```python
from build123d import *

# Parameters (mm, degrees)
SKETCH_1_R          = 21
SKETCH_1_R_2        = 10
EXTRUDE_1_DEPTH     = 36
SKETCH_1_R_3        = 16
EXTRUDE_1_2_DEPTH   = 36
SKETCH_2_W          = 150
SKETCH_2_H          = 5
EXTRUDE_3_DEPTH     = 5
SKETCH_3_W          = 150
SKETCH_3_H          = 5
EXTRUDE_4_DEPTH     = 5
EXTRUDE_5_DEPTH     = 5
EXTRUDE_START       = -3
SKETCH_7_R          = 16
EXTRUDE_7_DEPTH     = 30
SKETCH_8_R          = 0.9
CUT_EXTRUDE_1_DEPTH = 8
EXTRUDE_START_2     = -7
SKETCH_10_R         = 18.243216987
SKETCH_10_R_2       = 11
EXTRUDE_8_DEPTH     = 22


with BuildPart() as part:
    # Sketch 1 → Extrude 1 (new body)
    with BuildSketch(Plane(origin=(0, 0, 0), x_dir=(1, 0, 0), z_dir=(0, 1, 0))):
        with Locations((68.910572273, -5.294054995)):
            Circle(SKETCH_1_R)
        with Locations((68.910572273, -5.294054995)):
            Circle(SKETCH_1_R_2, mode=Mode.SUBTRACT)
    extrude(amount=EXTRUDE_1_DEPTH)



with BuildPart() as body_2:
    # Sketch 1 → Extrude 1 2 (new body)
    with BuildSketch(Plane(origin=(0, 0, 0), x_dir=(1, 0, 0), z_dir=(0, 1, 0))):
        with Locations((-81.089427727, -5.294054995)):
            Circle(SKETCH_1_R)
        with Locations((-81.089427727, -5.294054995)):
            Circle(SKETCH_1_R_3, mode=Mode.SUBTRACT)
    extrude(amount=EXTRUDE_1_2_DEPTH)


with BuildPart() as part_1:
    add(part.part)

    add(body_2.part)  # Extrude 3 merges body 2
    # Sketch 2 → Extrude 3 (add)
    with BuildSketch(Plane(origin=(0, 36, 0), x_dir=(1, 0, 0), z_dir=(0, 1, 0))):
        with Locations((-6.089427727, -23.794054995)):
            Rectangle(SKETCH_2_W, SKETCH_2_H)
        with Locations((-6.089427727, 13.205945005)):
            Rectangle(SKETCH_2_W, SKETCH_2_H)
    extrude(amount=-EXTRUDE_3_DEPTH)

    # Sketch 3 → Extrude 4 (add)
    with BuildSketch(Plane.XZ):
        with Locations((-6.089427727, -13.205945005)):
            Rectangle(SKETCH_3_W, SKETCH_3_H)
        with Locations((-6.089427727, 23.794054995)):
            Rectangle(SKETCH_3_W, SKETCH_3_H)
    extrude(amount=-EXTRUDE_4_DEPTH)

    # Sketch 4 → Extrude 5 (add)
    with BuildSketch(Plane.XZ):
        Polygon((-36.788692473, 8.113223678), (-7.244877213, 23.511020598), (-6.089427727, 21.294054995), (-4.933978242, 23.511020598), (24.609837018, 8.113223678), (54.153652279, 23.511020598), (56.46455125, 19.077089392), (30.018987378, 5.294054995), (56.46455125, -8.488979402), (54.153652279, -12.922910608), (24.609837018, 2.474886312), (-4.933978242, -12.922910608), (-7.244877213, -12.922910608), (-36.788692473, 2.474886312), (-66.332507733, -12.922910608), (-68.643406704, -8.488979402), (-42.197842833, 5.294054995), (-68.643406704, 19.077089392), (-66.332507733, 23.511020598), align=None)
        Polygon((-31.379542113, 5.294054995), (-8.589427727, -6.583813521), (-8.589427727, 17.17192351), align=None, mode=Mode.SUBTRACT)
        Polygon((-3.589427727, -6.583813521), (19.200686659, 5.294054995), (-3.589427727, 17.17192351), align=None, mode=Mode.SUBTRACT)
    extrude_5 = extrude(amount=-EXTRUDE_5_DEPTH)

    # Sketch 7 → Extrude 7 (add)
    with BuildSketch(Plane(origin=(0, 36, 0), x_dir=(1, 0, 0), z_dir=(0, 1, 0)).offset(EXTRUDE_START)):
        with Locations((68.910572273, -5.294054995)):
            Circle(SKETCH_7_R)
    extrude(amount=-EXTRUDE_7_DEPTH)

    # Sketch 8 → Cut-Extrude 1 (cut)
    with BuildSketch(Plane(origin=(0, 33, 0), x_dir=(1, 0, 0), z_dir=(0, 1, 0))):
        with Locations((76.910572273, -5.294054995)):
            Circle(SKETCH_8_R)
        with Locations((68.910572273, 2.705945005)):
            Circle(SKETCH_8_R)
        with Locations((74.567426522, 0.362799255)):
            Circle(SKETCH_8_R)
        with Locations((63.253718023, 0.362799255)):
            Circle(SKETCH_8_R)
        with Locations((60.910572273, -5.294054995)):
            Circle(SKETCH_8_R)
        with Locations((68.910572273, -13.294054995)):
            Circle(SKETCH_8_R)
        with Locations((63.253718023, -10.950909244)):
            Circle(SKETCH_8_R)
        with Locations((74.567426522, -10.950909244)):
            Circle(SKETCH_8_R)
    cut_extrude_1 = extrude(amount=-CUT_EXTRUDE_1_DEPTH, mode=Mode.SUBTRACT)

    # Mirror 1: Cut-Extrude 1 across plane
    add(cut_extrude_1.mirror(Plane.ZX.offset(18)), mode=Mode.SUBTRACT)

    # Mirror 2: Extrude 5 across plane
    add(extrude_5.mirror(Plane.ZX.offset(18)))

    # Sketch 10 → Extrude 8 (add)
    with BuildSketch(Plane(origin=(0, 36, 0), x_dir=(1, 0, 0), z_dir=(0, 1, 0)).offset(EXTRUDE_START_2)):
        with Locations((-81.089427727, -5.294054995)):
            Circle(SKETCH_10_R)
        with Locations((-81.089427727, -5.294054995)):
            Circle(SKETCH_10_R_2, mode=Mode.SUBTRACT)
    extrude(amount=-EXTRUDE_8_DEPTH)


solid = part_1.part
```
Here's how the part is built. I have some questions about the finished solid (model axes, mm). A direction names the side the tool comes from. Coordinates: 2 decimals unless noted, no trailing zeros. Loops run counter-clockwise (first coordinate to the right, second up) from the corner with the lowest first, then second, coordinate; pieces in that order, holes last. Notation, with made-up numbers: (65.25, 71.25) - (105.25, 71.25) arc R21 ccw to (105.25, 110.25) - close; hole circle Ø5 at (68.5, 76.5). An arc over 180 degrees is marked (long way). Return JSON: item names as keys, results as strings. Group by question number.
Item 1: On a 3-axis mill with a long thin cutter (end or side, diameter ignored), from which of +Z, -Z, +X, -X, +Y, -Y can I reach the whole of each face in a straight line? I mean faces 3 (the face through (-70.6, 29, 1.5)), 4 (the face through (17, 36, 10)), 5 (the face through (-37, 34, 21.294)). Say none if no direction works.
Item 2: If we section it at C-C on x = -33.5: Write out the boundary of the cut face in (y, z).
Item 3: Will these pins go through, and if not, where does the flat tip stop? P1, Ø0.9, axis at x = 77, z = 5.5, coming from the -Y side; P2, Ø4, axis at x = 15.5, y = 5.5, coming from the +Z side; P3, Ø2, axis at y = 24, z = 8, coming from the -X side; P4, Ø2, axis at x = 63.25, z = 10.95, coming from the +Y side.
Item 4: I need wall thicknesses on line 1 (Y direction, x = -33, z = 5); line 2 (Z direction, x = 13.5, y = 2); line 3 (Y direction, x = -68.5, z = -2). Which ranges of each line are inside material? Lowest first, please. Write a range as from..to.
Item 5: If we section it at B-B on x = 7: State how many separate pieces and enclosed holes the cut face has, and give its area (3 significant figures).
Item 6: If we section it at A-A on y = 18: Write out the boundary of the cut face in (x, z).
Item 7: If we section it at D-D on z = -13: Write out the boundary of the cut face in (x, y), and give its area (3 significant figures).
Item 8: We'd pull the mould along X, two halves only. Please class faces 1 (the face through (-5, 5, 6)), 2 (the face through (-7, 34, -15.706)): +X half, -X half, draft (parallel to the pull), parting line (faces both ways), or undercut.
Calculated:
{
 "1": {"face 3": "+Y", "face 4": "+Z, -Z, +X, -X, +Y", "face 5": "+Y, -Y"},
 "2": {"outline": "(0, -15.71) - (5, -15.71) - (5, -10.71) - (0, -10.71) - close; (0, 0.76) - (5, 0.76) - (5, 9.83) - (0, 9.83) - close; (0, 21.29) - (5, 21.29) - (5, 26.29) - (0, 26.29) - close; (31, -15.71) - (36, -15.71) - (36, -10.71) - (31, -10.71) - close; (31, 0.76) - (36, 0.76) - (36, 9.83) - (31, 9.83) - close; (31, 21.29) - (36, 21.29) - (36, 26.29) - (31, 26.29) - close"},
 "3": {"P1": "stops at y = 11", "P2": "stops at z = 26.29", "P3": "stops at x = -102.02", "P4": "stops at y = 33"},
 "4": {"line 1": "y = 0..5, 31..36", "line 2": "z = -15.71..-10.71, -3.32..2.32, 8.27..13.9, 21.29..26.29", "line 3": "y = 7..29"},
 "5": {"separate pieces": "8", "enclosed holes": "0", "area": "213 mm^2"},
 "6": {"outline": "circle Ø42 at (-81.09, 5.29); circle Ø42 at (68.91, 5.29); hole circle Ø22 at (-81.09, 5.29)"},
 "7": {"outline": "(-91.4, 0) - (79.22, 0) - (79.22, 36) - (-91.4, 36) - close; hole (-70.78, 5) - (58.6, 5) - (58.6, 31) - (-70.78, 31) - close", "area": "2,780 mm^2"},
 "8": {"face 1": "undercut", "face 2": "draft"}
}
